Geometry check sheet. Reference: the model listing, model coordinates, mm. Give positions to 0.01 mm unless a question says otherwise; leave off trailing zeros. Order: outer loops, then holes, each group sorted by start corner. A loop starts at its lowest first (then second) coordinate and runs counter-clockwise, first axis right, second up. Notation, with made-up numbers: M 6.25,-27 L 56.25,-27 A30 cw 56.25,12 Z; hole C 4,42 d4. An arc over 180 degrees is marked long. Put each result on its own line as item: value. Start each with the question number.
Q1. Material ranges on L1, parallel to Y at x = 0, z = 0.4; L2, parallel to X at y = 15, z = 1.4; L3, parallel to X at y = 17, z = 2.6, recorded low to high.
Q2. Section check D-D on z = 2. Record the cut outline in (x, y).
Q3. Section check C-C on y = -30. Record the cut outline in (x, z), then the cut area to 3 significant figures.
Q4. Section check A-A on x = 0. Record the cut outline in (y, z), then the cut area to 4 significant figures.
Q5. Go/stop test with flat-tipped pins: pin 1 (2 mm diameter, centred on y = 31.5, z = 1.5, fed in from +X); pin 2 (12 mm diameter, centred on x = -7.5, y = -2, fed in from +Z); pin 3 (3 mm diameter, centred on y = -30.5, z = 2.5, fed in from +X); pin 4 (5 mm diameter, centred on x = 0, y = -30, fed in from +Z). Record where each tip stops, or that it passes through.
Q6. Section check B-B on y = 15. Record the cut outline in (x, z).
Q7. Mould release check, pull along Y, two halves, no side actions. Record for faces 1 (the flat face through (0, 0, 4)), 2 (the cylindrical face through (-28.604, 14.174, 2.535)), 3 (the flat face through (26, 1, 5)), 4 (the cylindrical face through (-8.67, -39.05, 2.46)): +Y half, -Y half, draft (parallel to the pull), parting line (faces both ways), or undercut.
```python
from build123d import *

# Parameters (mm, degrees)
F0_R     = 40
F1_DEPTH = 5
F2_W     = 40
F2_H     = 41
F3_DEPTH = 1
F5_D     = 5.5
F6_DEPTH = 1


with BuildPart() as f1:
    # F0 (on Top) → F1 (new body)
    with BuildSketch(Plane.XY):
        Circle(F0_R)
    extrude(amount=F1_DEPTH)

    # F2 (on face) → F3 (cut)
    with BuildSketch(Plane.XY.offset(5)):
        Rectangle(F2_W, F2_H)
    extrude(amount=-F3_DEPTH, mode=Mode.SUBTRACT)

    # F5 (through all)
    with Locations(Plane(origin=(0, 0, 0), x_dir=(1, 0, 0), z_dir=(0, 0, -1))):
        with Locations((0, 30), (25.980762, -15), (-25.980762, -15)):
            Hole(F5_D / 2)

    # F2 (on face) → F6 (cut)
    with BuildSketch(Plane.XY.offset(5)):
        Rectangle(F2_W, F2_H)
    extrude(amount=-F6_DEPTH, mode=Mode.SUBTRACT)


solid = f1.part
```
Results found:
1. L1: y = -40 to -32.75, -27.25 to 40
1. L2: x = -37.08 to -28.73, -23.23 to 23.23, 28.73 to 37.08
1. L3: x = -36.21 to -27.87, -24.09 to 24.09, 27.87 to 36.21
2. outline: C 0,0 d80; hole C -25.98,15 d5.5; hole C 0,-30 d5.5; hole C 25.98,15 d5.5
3. outline: M -26.46,0 L -2.75,0 L -2.75,5 L -26.46,5 Z; M 2.75,0 L 26.46,0 L 26.46,5 L 2.75,5 Z
3. area: 237 mm^2
4. outline: M -40,0 L -32.75,0 L -32.75,5 L -40,5 Z; M -27.25,0 L 40,0 L 40,5 L 20.5,5 L 20.5,4 L -20.5,4 L -20.5,5 L -27.25,5 Z
4. area: 331.5 mm^2
5. pin 1: stops at x = 25.88
5. pin 2: stops at z = 4
5. pin 3: stops at x = 27.55
5. pin 4: passes through
6. outline: M -37.08,0 L -28.73,0 L -28.73,5 L -37.08,5 Z; M -23.23,0 L 23.23,0 L 23.23,5 L 20,5 L 20,4 L -20,4 L -20,5 L -23.23,5 Z; M 28.73,0 L 37.08,0 L 37.08,5 L 28.73,5 Z
7. face 1: undercut
7. face 2: undercut
7. face 3: draft
7. face 4: parting line
